The listing builds one solid part. Answer for the finished solid, in the listing's coordinates (mm). A direction names the side the tool comes from. Give positions to 0.01 mm unless a question says otherwise; leave off trailing zeros. Loops run counter-clockwise (first coordinate to the right, second up) from the corner with the lowest first, then second, coordinate; pieces in that order, holes last. Notation, with made-up numbers: M 23,57.25 L 32,57.25 A7 cw 32,68.25 Z; hole C 85,-0.75 d4. An arc over 180 degrees is marked long. Return JSON: item names as keys, results as strings.
from build123d import *

# Parameters (mm, degrees)
RESSALTO_EXTRUS_O1_DEPTH = 5.55


with BuildPart() as part:
    # Esboço1 → Ressalto-extrusão1 (new body)
    with BuildSketch(Plane.XY):
        with BuildLine():
            Line((-15.5, -28.119565217), (15.5, -28.119565217))
            ThreePointArc((15.5, -28.119565217), (18.328427125, -29.291138093), (19.5, -32.119565217))
            Line((19.5, -32.119565217), (19.5, -40.619565217))
            ThreePointArc((19.5, -40.619565217), (22.534152087, -44.501206341), (27.033568905, -42.494102706))
            Line((27.033568905, -42.494102706), (32.73188308, -31.75258065))
            ThreePointArc((32.73188308, -31.75258065), (33.428027517, -29.935201499), (33.664745271, -28.003505673))
            Line((33.664745271, -28.003505673), (33.664745271, -24.494102706))
            ThreePointArc((33.664745271, -24.494102706), (37.669109742, -2.578069762), (49.164745271, 16.505897294))
            ThreePointArc((49.164745271, 16.505897294), (49.287222325, 23.539892597), (42.362401343, 24.780434783))
            Line((42.362401343, 24.780434783), (15.046868421, 8.983444446))
            ThreePointArc((15.046868421, 8.983444446), (14.322494504, 8.682938362), (13.544989202, 8.580434783))
            Line((13.544989202, 8.580434783), (-13.544989202, 8.580434783))
            ThreePointArc((-13.544989202, 8.580434783), (-14.322494504, 8.682938362), (-15.046868421, 8.983444446))
            Line((-15.046868421, 8.983444446), (-42.362401343, 24.780434783))
            ThreePointArc((-42.362401343, 24.780434783), (-49.287222325, 23.539892597), (-49.164745271, 16.505897294))
            ThreePointArc((-49.164745271, 16.505897294), (-37.669109742, -2.578069762), (-33.664745271, -24.494102706))
            Line((-33.664745271, -24.494102706), (-33.664745271, -28.003505673))
            ThreePointArc((-33.664745271, -28.003505673), (-33.428027517, -29.935201499), (-32.73188308, -31.75258065))
            Line((-32.73188308, -31.75258065), (-27.033568905, -42.494102706))
            ThreePointArc((-27.033568905, -42.494102706), (-22.534152087, -44.501206341), (-19.5, -40.619565217))
            Line((-19.5, -40.619565217), (-19.5, -32.119565217))
            ThreePointArc((-19.5, -32.119565217), (-18.328427125, -29.291138093), (-15.5, -28.119565217))
        make_face()
    extrude(amount=RESSALTO_EXTRUS_O1_DEPTH)


solid = part.part
(1) The part is cut by section C-C (x = -10.5). Determine the outline of the cut face in (y, z), and give its area (3 significant figures).
Values follow:
{"outline": "M -28.12,0 L 8.58,0 L 8.58,5.55 L -28.12,5.55 Z", "area": "204 mm²"}
(2) The part is cut by section D-D (y = -16). Determine the outline of the cut face in (x, z).
Values follow:
{"outline": "M -34.25,0 L 34.25,0 L 34.25,5.55 L -34.25,5.55 Z"}
(3) Determine the mould class of faces 6 (the cylindrical face through (-22.61, -44.52, 2.74)), 7 (the cylindrical face through (-33.435, -29.909, 2.736)), 8 (the cylindrical face through (37.56, -2.87, 2.74)) for opening direction X: released by +X, released by -X, zero draft, split by the parting line, or undercut.
Values follow:
{"face 6": "undercut", "face 7": "released by -X", "face 8": "released by +X"}
(4) A tool of negligible diameter and unlimited length cuts with its end or side. For faces 1 (the flat face through (33.665, -26, 3)), 2 (the flat face through (-1, -9, 5.55)), 3 (the flat face through (0, 8.58, 3)), 4 (the cylindrical face through (-49.22, 23.62, 2.74)), 5 (the flat face through (19.5, -36, 3)), from which of +Z, -Z, +X, -X, +Y, -Y can it reach the whole face along a straight path? Write none if from no direction.
Values follow:
{"face 1": "+Z, -Z, +X, -Y", "face 2": "+Z, +X, -X, +Y, -Y", "face 3": "+Z, -Z, +Y", "face 4": "+Z, -Z", "face 5": "+Z, -Z, -Y"}
(5) The part is cut by section A-A (y = 21). Determine the outline of the cut face in (x, z).
Values follow:
{"outline": "M -50.45,0 L -35.83,0 L -35.83,5.55 L -50.45,5.55 Z; M 35.83,0 L 50.45,0 L 50.45,5.55 L 35.83,5.55 Z"}
(6) Straight lines are drawn through the part: line 1 along Y through (x, z) = (-6.5, 3.65); line 2 along X through (y, z) = (-33, 5.35); line 3 along X through (y, z) = (-30, 4.45). For each, find the intervals that lie inside material, in ascending order.
Values follow:
{"line 1": "-28.12 to 8.58", "line 2": "-32.07 to -19.5, 19.5 to 32.07", "line 3": "-33.41 to -18.89, 18.89 to 33.41"}
(7) Given pin 1 (3 mm diameter, centred on x = 24.5, z = 3, fed in from -Y); pin 2 (3 mm diameter, centred on x = -0.5, z = 1.5, fed in from +Y); pin 3 (3 mm diameter, centred on x = -29, z = 2.5, fed in from -Y); pin 4 (1 mm diameter, centred on x = -38, z = 2, fed in from +Y), each flat-ended and moving along its own axis, determine where each tip first touches the part or whether it passes through.
Values follow:
{"pin 1": "y = -44.62", "pin 2": "y = 8.58", "pin 3": "y = -41.61", "pin 4": "y = 22.55"}
